For this review, use the dimensioned drawing (mm, ordinates from the lowest corner) and the shaded views. Give positions to 0.01 mm unless a question says otherwise; leave off trailing zeros. Order: outer loops, then holes, each group sorted by start corner. A loop starts at its lowest first (then second) coordinate and runs counter-clockwise, first axis right, second up. Notation, with made-up numbers: (84.5, 74) -> (107.5, 74) arc R27 ccw to (107.5, 101) -> close; hole circle Ø2 at (80, 49). An arc over 180 degrees is marked (long way). One line per item, written item: value. Start each with the question number.
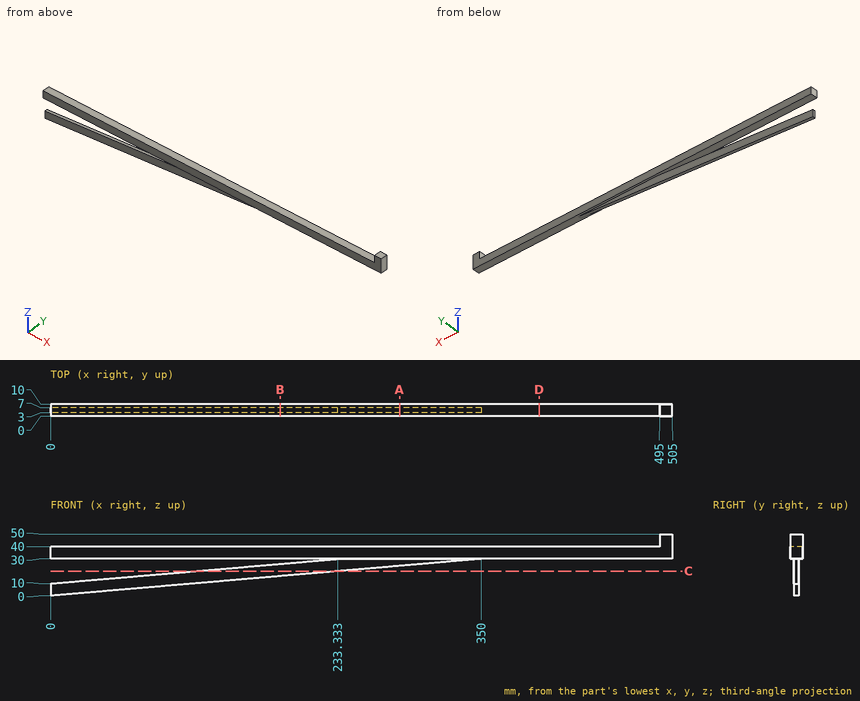
Q1. For pin 1 Ø15 at (x, z) = (183, 17) entering from -Y; pin 2 Ø24 at (x, z) = (255.5, 13.5) entering from +Y; pin 3 Ø2 at (x, y) = (247.5, 3.5) entering from -Z, all flat-tipped, find the tip position at first contact; note any pin that passes through.
Q2. Take a section at B-B (x = 186.5). State the section outline as (y, z) points, and give its area (3 significant figures).
Q3. For line 1 along Z through (x, y) = (188.5, 8.25); line 2 along Y through (x, z) = (141.5, 22); line 3 along X through (y, z) = (2.5, 47), list the stretches that pass through material, from the lowest coordinate up.
Q4. Take a section at A-A (x = 283.5). State the section outline as (y, z) points.
Q5. Take a section at C-C (z = 20). State the section outline as (x, y) points, and give its area (3 significant figures).
Q6. Take a section at D-D (x = 397). State the section outline as (y, z) points, and give its area (3 significant figures).
Answers below:
1. pin 1: stops at y = 3
1. pin 2: stops at y = 7
1. pin 3: stops at z = 21.13
2. outline: (0, 30) -> (10, 30) -> (10, 40) -> (0, 40) -> close; (3, 15.99) -> (7, 15.99) -> (7, 25.99) -> (3, 25.99) -> close
2. area: 140 mm²
3. line 1: z = 30 to 40
3. line 2: y = 3 to 7
3. line 3: x = 495 to 505
4. outline: (0, 30) -> (3, 30) -> (3, 24.3) -> (7, 24.3) -> (7, 30) -> (10, 30) -> (10, 40) -> (0, 40) -> close
5. outline: (116.67, 3) -> (233.33, 3) -> (233.33, 7) -> (116.67, 7) -> close
5. area: 467 mm²
6. outline: (0, 30) -> (10, 30) -> (10, 40) -> (0, 40) -> close
6. area: 100 mm²
